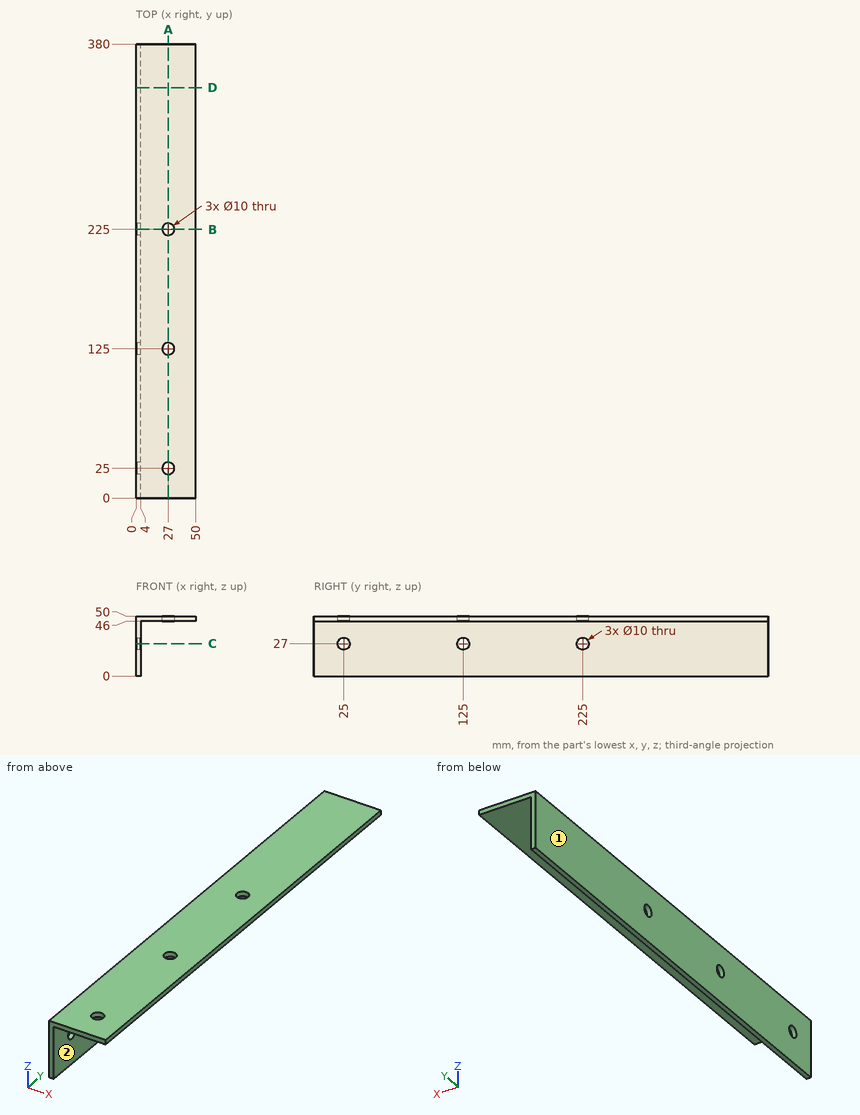
Geometry check sheet. Reference: drawing and pictorial views, mm from the part's lowest x, y, z. A direction names the side the tool comes from. Give positions to 0.01 mm unless a question says otherwise; leave off trailing zeros. Write each loop counter-clockwise with the first axis right and the second up, starting at its lowest first coordinate (ties: lowest second). Pieces come first, ordered by that corner, then holes. Notation, with made-up numbers: M 18,89 L 34,89 A30 ccw 34,116 Z; hole C 59.5,61 d5. An arc over 180 degrees is marked long. Use CSV: the item, a comma, the result in double quotes.
1) Cross-section at A-A (x = 27). Enter the section's corners in (y, z), plus the area to 3 significant figures.
Final values:
outline,"M 0,46 L 20,46 L 20,50 L 0,50 Z; M 30,46 L 120,46 L 120,50 L 30,50 Z; M 130,46 L 220,46 L 220,50 L 130,50 Z; M 230,46 L 380,46 L 380,50 L 230,50 Z"
area,"1,400 mm²"
2) Access from +Z, -Z, +X, -X, +Y, -Y to the whole of each face (thin tool, end or side, straight path). Record for the marked faces 1 and 2.
Final values:
face 1,"+Z, -Z, -X, +Y, -Y"
face 2,"-Z, +X, +Y, -Y"
3) Cross-section at D-D (y = 343.5). Enter the section's corners in (x, z), plus the area to 3 significant figures.
Final values:
outline,"M 0,0 L 4,0 L 4,46 L 50,46 L 50,50 L 0,50 Z"
area,"384 mm²"
4) Material ranges on line 1 along Y through (x, z) = (2, 27); line 2 along Z through (x, y) = (25, 68); line 3 along X through (y, z) = (195.5, 38), recorded low to high.
Final values:
line 1,"0 to 20, 30 to 120, 130 to 220, 230 to 380"
line 2,"46 to 50"
line 3,"0 to 4"
5) Cross-section at C-C (z = 27). Enter the section's corners in (x, y).
Final values:
outline,"M 0,0 L 4,0 L 4,20 L 0,20 Z; M 0,30 L 4,30 L 4,120 L 0,120 Z; M 0,130 L 4,130 L 4,220 L 0,220 Z; M 0,230 L 4,230 L 4,380 L 0,380 Z"
6) Cross-section at B-B (y = 225). Enter the section's corners in (x, z), plus the area to 3 significant figures.
Final values:
outline,"M 0,0 L 4,0 L 4,22 L 0,22 Z; M 0,32 L 4,32 L 4,46 L 22,46 L 22,50 L 0,50 Z; M 32,46 L 50,46 L 50,50 L 32,50 Z"
area,"304 mm²"
7) Go/stop test with flat-tipped pins: pin 1 Ø12 at (y, z) = (290, 25.5) entering from +X; pin 2 Ø13 at (y, z) = (225, 27) entering from -X; pin 3 Ø8 at (x, y) = (27, 125) entering from +Z; pin 4 Ø23 at (x, y) = (26.5, 256) entering from -Z. Record where each tip stops, or that it passes through.
Final values:
pin 1,"x = 4"
pin 2,"x = 0"
pin 3,"through"
pin 4,"z = 46"
